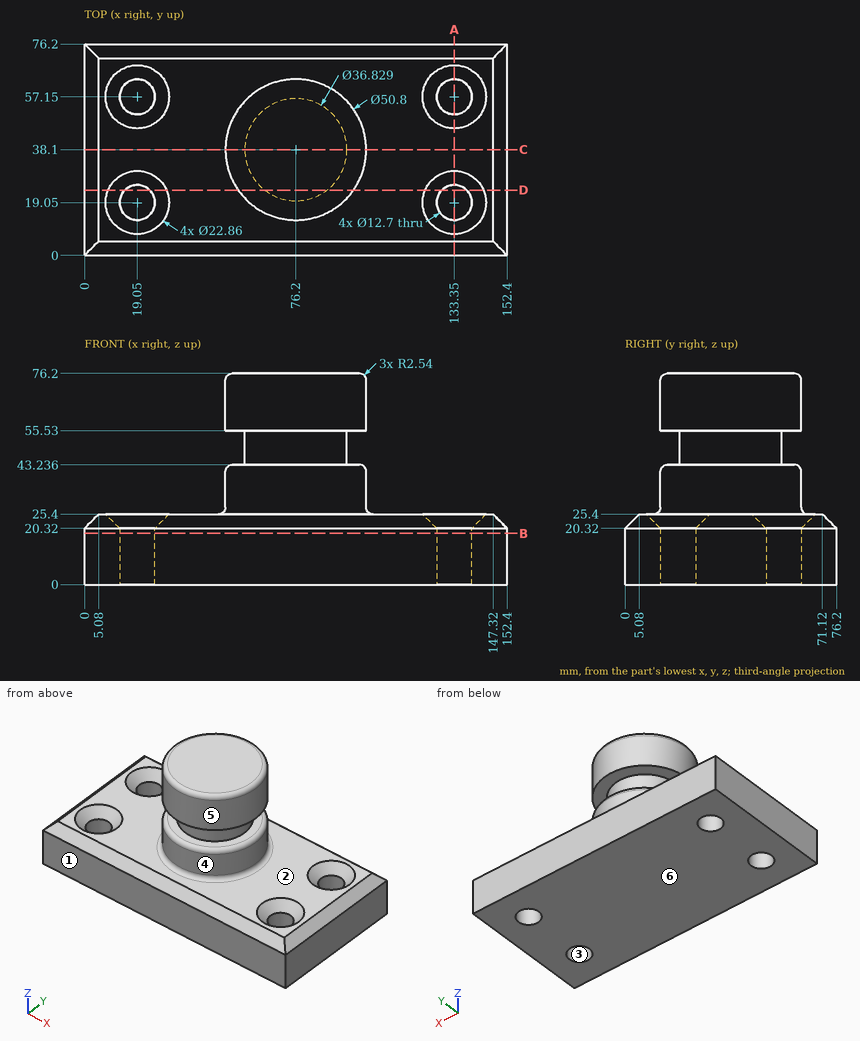
Here's the drawing with two shaded views (mm, measured from the low corner). I have some questions. A direction names the side the tool comes from. Coordinates: 2 decimals unless noted, no trailing zeros. Loops run counter-clockwise (first coordinate to the right, second up) from the corner with the lowest first, then second, coordinate; pieces in that order, holes last. Notation, with made-up numbers: M 22.25,-33 L 39.25,-33 A25 cw 39.25,-2 Z; hole C 63,35 d7. An arc over 180 degrees is marked long. Put each result on its own line as item: value. Start each with the question number.
(1) Which directions (+Z, -Z, +X, -X, +Y, -Y) give clear straight access to the entire face, cutting with the end or side of a thin tool? Please do the marked faces 5 and 6.
(2) Imagine slicing it at B-B on z = 18.5. List the corners of the cut face in (x, y) for me.
(3) I need wall thicknesses on probe 1 along Y at (x, z) = (133, 9); probe 2 along X at (y, z) = (19, 8); probe 3 along Z at (x, y) = (71, 57). Which ranges of each line are inside material? Lowest first, please.
(4) We'd pull the mould along Y, two halves only. Please class the marked faces 1, 2, 3 and 4: +Y half, -Y half, draft (parallel to the pull), parting line (faces both ways), or undercut.
(5) Imagine slicing it at D-D on y = 23.5. Give the number of separate pieces and of enclosed holes in the cut face.
(6) Will these pins go through, and if not, where does the flat tip stop? pin 1 Ø7.5 at (x, y) = (19.05, 57.15) entering from +Z; pin 2 Ø4 at (x, y) = (20, 32.5) entering from +Z; pin 3 Ø20.5 at (x, y) = (133.35, 19.05) entering from +Z; pin 4 Ø6 at (y, z) = (58.5, 36) entering from +X (1 decimal).
(7) Imagine slicing it at C-C on y = 38.1. List the corners of the cut face in (x, z) for me (1 decimal), and give its area (3 significant figures).
(8) Imagine slicing it at A-A on x = 133.35. List the corners of the cut face in (y, z) for me.
Worked answers:
1. face 5: +Z
1. face 6: -Z, +X, -X, +Y, -Y
2. outline: M 0,0 L 152.4,0 L 152.4,76.2 L 0,76.2 Z; hole C 19.05,19.05 d12.7; hole C 19.05,57.15 d12.7; hole C 133.35,19.05 d12.7; hole C 133.35,57.15 d12.7
3. probe 1: y = 0 to 12.71, 25.39 to 50.81, 63.49 to 76.2
3. probe 2: x = 0 to 12.7, 25.4 to 127, 139.7 to 152.4
3. probe 3: z = 0 to 43.24, 55.53 to 76.2
4. face 1: -Y half
4. face 2: draft
4. face 3: undercut
4. face 4: parting line
5. separate pieces: 3
5. enclosed holes: 0
6. pin 1: passes through
6. pin 2: stops at z = 25.4
6. pin 3: stops at z = 24.22
6. pin 4: stops at x = 94.7
7. outline: M 0,0 L 152.4,0 L 152.4,20.3 L 147.3,25.4 L 104.1,25.4 A2.5 cw 101.6,27.9 L 101.6,40.7 A2.5 ccw 99.1,43.2 L 94.6,43.2 L 94.6,55.5 L 101.6,55.5 L 101.6,73.7 A2.5 ccw 99.1,76.2 L 53.3,76.2 A2.5 ccw 50.8,73.7 L 50.8,55.5 L 57.8,55.5 L 57.8,43.2 L 53.3,43.2 A2.5 ccw 50.8,40.7 L 50.8,27.9 A2.5 cw 48.3,25.4 L 5.1,25.4 L 0,20.3 Z
7. area: 6,250 mm2
8. outline: M 0,0 L 12.7,0 L 12.7,20.32 L 7.62,25.4 L 5.08,25.4 L 0,20.32 Z; M 25.4,0 L 50.8,0 L 50.8,20.32 L 45.72,25.4 L 30.48,25.4 L 25.4,20.32 Z; M 63.5,0 L 76.2,0 L 76.2,20.32 L 71.12,25.4 L 68.58,25.4 L 63.5,20.32 Z
